Autodesk Inventor part; units mm, degrees
ref_plane "Arbeitsebene1" through (0, 0, 11) normal (0, 0, 1) x (1, 0, 0)
ref_plane "YZ Plane" through (0, 0, 0) normal (1, 0, 0) x (0, 1, 0)
ref_plane "XZ Plane" through (0, 0, 0) normal (0, 1, 0) x (-1, 0, 0)
sketch "Skizze1" plane through (0, 0, 0) normal (1, 0, 0) x (0, 1, 0)
  circle A0 centre (0, 0) radius 11
  dimension "d0" = 22
extrude "Extrusion1" add sketch "Skizze1" along normal blind 191
shell "Wandung1" thickness 1.5 removed faces 1 at (0, -3.2467, -1.704)
ref_plane "Arbeitsebene1" through (0, 0, 11) normal (0, 0, 1) x (1, 0, 0)
sketch "Skizze2" plane through (0, 0, 11) normal (0, 0, 1) x (1, 0, 0)
  circle A0 centre (106, 0) radius 9
  circle A1 centre (141, 0) radius 9
  circle A2 centre (176, 0) radius 9
  line L0 (191, -11) -> (191, 11)
  line L1 (0, -11) -> (0, 11)
  point P0 (0, 0)
  dimension "d6" = 15
  dimension "d7" = 35
  dimension "d8" = 35
  dimension "d9" = 18
extrude "Extrusion2" cut sketch "Skizze2" against normal blind 6
properties part number "102 part 2" material "Aluminum 6061, geschweißt"
Geometry check sheet. Reference: the model listing, model coordinates, mm. A direction names the side the tool comes from. Give positions to 0.01 mm unless a question says otherwise; leave off trailing zeros. Order: outer loops, then holes, each group sorted by start corner. A loop starts at its lowest first (then second) coordinate and runs counter-clockwise, first axis right, second up. Notation, with made-up numbers: (22, 82.5) - (54, 82.5) arc R21 cw to (54, 100.5) - close; hole circle Ø5 at (63.5, 28.5). An arc over 180 degrees is marked (long way). Answer as a JSON object with one key per item and string values.
(1) Cross-section at D-D (z = -7). Record the cut outline in (x, y), then the cut area to 3 significant figures.
Report:
{"outline": "(0, -8.49) - (191, -8.49) - (191, 8.49) - (0, 8.49) - (0, 6.42) - (189.5, 6.42) - (189.5, -6.42) - (0, -6.42) - close", "area": "807 mm^2"}
(2) Cross-section at B-B (z = 0). Record the cut outline in (x, y).
Report:
{"outline": "(0, -11) - (191, -11) - (191, 11) - (0, 11) - (0, 9.5) - (189.5, 9.5) - (189.5, -9.5) - (0, -9.5) - close"}
(3) Cross-section at C-C (x = 25.5). Record the cut outline in (y, z).
Report:
{"outline": "circle Ø22 at (0, 0); hole circle Ø19 at (0, 0)"}
(4) Material ranges on line 1 (X direction, y = 0, z = 7.5); line 2 (Z direction, x = 23, y = -0.25); line 3 (Y direction, x = 66.5, z = -0.75), recorded low to high.
Report:
{"line 1": "189.5 to 191", "line 2": "-11 to -9.5, 9.5 to 11", "line 3": "-10.97 to -9.47, 9.47 to 10.97"}
(5) Draft check along Y on faces 4 (the flat face through (0, -10, 0)), 5 (the cylindrical face through (182.271, 6.455, 8.015)), 6 (the cylindrical face through (94.163, -1.432, -10.906)). Enter one of: released by +Y, released by -Y, zero draft, split by the parting line, or undercut.
Report:
{"face 4": "zero draft", "face 5": "undercut", "face 6": "split by the parting line"}
(6) Cross-section at A-A (y = -1.75). Record the cut outline in (x, z).
Report:
{"outline": "(0, -10.86) - (191, -10.86) - (191, 10.86) - (184.83, 10.86) - (184.83, 9.34) - (189.5, 9.34) - (189.5, -9.34) - (0, -9.34) - close; (0, 9.34) - (97.17, 9.34) - (97.17, 10.86) - (0, 10.86) - close; (114.83, 9.34) - (132.17, 9.34) - (132.17, 10.86) - (114.83, 10.86) - close; (149.83, 9.34) - (167.17, 9.34) - (167.17, 10.86) - (149.83, 10.86) - close"}
(7) Tool access check on faces 1 (the cylindrical face through (93.42, -1.24, -9.42)), 2 (the flat face through (191, 0, 0)), 3 (the cylindrical face through (147.271, 6.455, 8.015)). Record the directions out of +Z, -Z, +X, -X, +Y, -Y that give a thin tool (end or side, any length) a straight path to the whole face; none if there is none.
Report:
{"face 1": "-X", "face 2": "+Z, -Z, +X, +Y, -Y", "face 3": "+Z"}
(8) Depth check by flat-ended pin: pin 1 Ø1 at (x, z) = (111, -3.5) entering from -Y; pin 2 Ø6 at (x, z) = (103, 1.5) entering from -Y; pin 3 Ø2 at (x, z) = (111, 5.5) entering from +Y; pin 4 Ø6 at (y, z) = (3, 4) entering from -X. Enter the tip coordinate at first touch or a pass-through.
Report:
{"pin 1": "y = -10.58", "pin 2": "y = -11", "pin 3": "y = 10.04", "pin 4": "x = 189.5"}
